Could you check a few things on this model? Use its own coordinates, in mm. A direction names the side the tool comes from. Coordinates: 2 decimals unless noted, no trailing zeros. Write each loop counter-clockwise with the first axis right and the second up, starting at its lowest first coordinate (ties: lowest second). Pieces come first, ordered by that corner, then holes. Notation, with made-up numbers: M 14.5,64.25 L 65.5,64.25 A9 ccw 65.5,81.25 Z; hole C 12.25,-25.75 d6. An arc over 180 degrees is marked long. Answer as CSV lines item,"result". Start each with the question number.
Item 1: I'm going to push flat-ended pins straight in: P1, Ø6.5, axis at x = 14, z = 13.5, coming from the +Y side (3 decimals); P2, Ø6, axis at y = 12, z = 6.5, coming from the +X side (3 decimals); P3, Ø1, axis at y = 16, z = 4.5, coming from the -X side; P4, Ø4, axis at y = 19.05, z = 12.7, coming from the -X side. Where does each tip first touch, or does it pass through?
Item 2: Suppose I cut it at C-C, the plane z = 12.7. Write out the boundary of the cut face in (x, y) (3 decimals).
Item 3: On a 3-axis mill with a long thin cutter (end or side, diameter ignored), from which of +Z, -Z, +X, -X, +Y, -Y can I reach the whole of each face in a straight line? I mean faces 5 (the cylindrical face through (6.224, 1.61, 12.775)), 6 (the flat face through (7, 2, 0)), 7 (the flat face through (14, 3.175, 7)). Say none if no direction works.
Item 4: We'd pull the mould along X, two halves only. Please class faces 1 (the flat face through (15, 2, 9.271)), 2 (the flat face through (3.175, 14, 13)), 3 (the flat face through (0, 13, 13)), 4 (the flat face through (13, 0, 7)): +X half, -X half, draft (parallel to the pull), parting line (faces both ways), or undercut.
Item 5: Suppose I cut it at D-D, the plane z = 18.75. Write out the boundary of the cut face in (x, y) (3 decimals), and give its area (3 significant figures).
Item 6: Suppose I cut it at A-A, the plane y = 19.05. Write out the boundary of the cut face in (x, z) (3 decimals), and give its area (3 significant figures).
Item 7: If I drill on line 1 along Y through (x, z) = (2.35, 12.7); line 2 along X through (y, z) = (15.25, 3.5) (3 decimals), over which ranges is the centre line in solid material (lowest first)? Write a range as [from, to].
Item 8: Suppose I cut it at B-B, the plane x = 12. Write out the boundary of the cut face in (y, z) (3 decimals), and give its area (3 significant figures).
```python
from build123d import *

# Parameters (mm, degrees)
BOSS_EXTRUDE1_DEPTH = 25.4
CUT_EXTRUDE1_DEPTH  = 25.4
SKETCH3_R           = 3.3734375
CUT_EXTRUDE2_DEPTH  = 25.4


with BuildPart() as part:
    # Sketch1 → Boss-Extrude1 (new body)
    with BuildSketch(Plane.XY):
        Polygon((0, 0), (0, 25.4), (3.175, 25.4), (3.175, 3.175), (25.4, 3.175), (25.4, 0), align=None)
    extrude(amount=BOSS_EXTRUDE1_DEPTH)

    # Sketch2 → Cut-Extrude1 (cut)
    with BuildSketch(Plane(origin=(0, 3.175, 0), x_dir=(1, 0, 0), z_dir=(0, 1, 0))):
        with BuildLine():
            Line((9.652, -9.271), (19.558, -9.271))
            ThreePointArc((19.558, -9.271), (22.987, -12.7), (19.558, -16.129))
            Line((19.558, -16.129), (9.652, -16.129))
            ThreePointArc((9.652, -16.129), (6.223, -12.7), (9.652, -9.271))
        make_face()
    extrude(amount=-CUT_EXTRUDE1_DEPTH, mode=Mode.SUBTRACT)

    # Sketch3 → Cut-Extrude2 (cut)
    with BuildSketch(Plane(origin=(3.175, 0, 0), x_dir=(0, 0, -1), z_dir=(1, 0, 0))):
        with Locations((-12.7, 19.05)):
            Circle(SKETCH3_R)
    extrude(amount=-CUT_EXTRUDE2_DEPTH, mode=Mode.SUBTRACT)


solid = part.part
```
Ans:
1,P1,"stops at y = 3.175"
1,P2,"stops at x = 3.175"
1,P3,"stops at x = 0"
1,P4,"passes through"
2,outline,"M 0,0 L 6.223,0 L 6.223,3.175 L 3.175,3.175 L 3.175,15.677 L 0,15.677 Z; M 0,22.423 L 3.175,22.423 L 3.175,25.4 L 0,25.4 Z; M 22.987,0 L 25.4,0 L 25.4,3.175 L 22.987,3.175 Z"
3,face 5,"+Y, -Y"
3,face 6,"-Z, +X, -X, +Y, -Y"
3,face 7,"+Z, -Z, +X, +Y"
4,face 1,"undercut"
4,face 2,"+X half"
4,face 3,"-X half"
4,face 4,"draft"
5,outline,"M 0,0 L 25.4,0 L 25.4,3.175 L 3.175,3.175 L 3.175,25.4 L 0,25.4 Z"
5,area,"151 mm^2"
6,outline,"M 0,0 L 3.175,0 L 3.175,9.327 L 0,9.327 Z; M 0,16.073 L 3.175,16.073 L 3.175,25.4 L 0,25.4 Z"
6,area,"59.2 mm^2"
7,line 1,"y = [0, 15.68], [22.42, 25.4]"
7,line 2,"x = [0, 3.175]"
8,outline,"M 0,0 L 3.175,0 L 3.175,9.271 L 0,9.271 Z; M 0,16.129 L 3.175,16.129 L 3.175,25.4 L 0,25.4 Z"
8,area,"58.9 mm^2"
